```python
from build123d import *

# Parameters (mm, degrees)
SKETCH2_R           = 1.4
SKETCH2_R_2         = 2.5
BOSS_EXTRUDE1_DEPTH = 4
BOSS_EXTRUDE2_START = 16.8
SKETCH3_R           = 4.65
SKETCH3_R_2         = 2.5
BOSS_EXTRUDE2_DEPTH = 16.8
SKETCH5_R           = 4.65
SKETCH5_R_2         = 2.5
BOSS_EXTRUDE3_DEPTH = 2
FILLET1_R           = 2
RIB1_REACH          = 36.514
SKETCH6_WALL_W      = 80.220281068
SKETCH6_WALL_H      = 1.6


with BuildPart() as part:
    # Sketch2 → Boss-Extrude1 (new body)
    with BuildSketch(Plane(origin=(0, 0, 0), x_dir=(1, 0, 0), z_dir=(0, 1, 0))):
        with BuildLine():
            Line((-9.4, -4.65), (0, -4.65))
            ThreePointArc((0, -4.65), (3.288046533, -3.288046533), (4.65, 0))
            Line((4.65, 0), (4.65, 22.6))
            ThreePointArc((4.65, 22.6), (0, 27.25), (-4.65, 22.6))
            Line((-4.65, 22.6), (-4.65, 2.35))
            Line((-4.65, 2.35), (-9.4, 2.35))
            ThreePointArc((-9.4, 2.35), (-12.9, -1.15), (-9.4, -4.65))
        make_face()
        with Locations(Location((-9.4, -1.15, 0), (0, 0, 270))):
            Circle(SKETCH2_R, mode=Mode.SUBTRACT)
        with Locations(Location((0, -1.15, 0), (0, 0, 270))):
            Circle(SKETCH2_R, mode=Mode.SUBTRACT)
        with Locations(Location((0, 22.6, 0), (0, 0, 270))):
            Circle(SKETCH2_R_2, mode=Mode.SUBTRACT)
    extrude(amount=BOSS_EXTRUDE1_DEPTH)

    # Sketch3 → Boss-Extrude2 (add)
    with BuildSketch(Plane.XZ.offset(BOSS_EXTRUDE2_START)):
        with Locations((0, -22.6)):
            Circle(SKETCH3_R)
        with Locations(Location((0, -22.6, 0), (0, 0, 90))):
            Circle(SKETCH3_R_2, mode=Mode.SUBTRACT)
    extrude(amount=-BOSS_EXTRUDE2_DEPTH)

    # Sketch5 → Boss-Extrude3 (add)
    with BuildSketch(Plane(origin=(0, 4, 0), x_dir=(1, 0, 0), z_dir=(0, 1, 0))):
        with Locations(Location((0, 22.6, 0), (0, 0, 270))):
            Circle(SKETCH5_R)
        with Locations(Location((0, 22.6, 0), (0, 0, 270))):
            Circle(SKETCH5_R_2, mode=Mode.SUBTRACT)
    extrude(amount=BOSS_EXTRUDE3_DEPTH)

    # Fillet1
    fillet1_edges = [part.edges().sort_by_distance(p)[0] for p in [
        (0, 6, -27.25),
    ]]
    fillet(fillet1_edges, radius=FILLET1_R - 0.0001)  # a hair under: the kernel refuses the full size

    # Sketch6 wall → Rib1 (add, up to next)
    with BuildSketch(Plane(origin=(0, -3.25, -14.7), x_dir=(0, -0.707106781187, -0.707106781187), z_dir=(0, 0.707106781187, -0.707106781187)), mode=Mode.PRIVATE) as rib1_sk1:
        Rectangle(SKETCH6_WALL_W, SKETCH6_WALL_H)
    rib1_tool1 = extrude(rib1_sk1.sketch, amount=RIB1_REACH, mode=Mode.PRIVATE) - part.part
    add(rib1_tool1.solids().sort_by_distance((0, -3.25, -14.7))[0])


solid = part.part
```
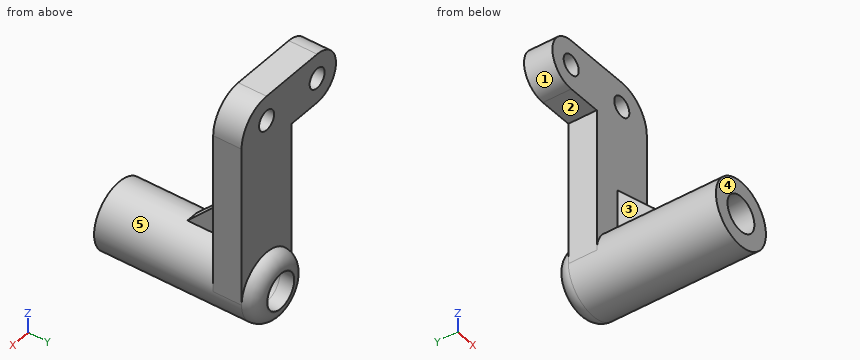
For this review, take the finished solid that the model builds, in its own axes (mm). Face numbers are marked on the shaded views. A direction names the side the tool comes from. Round coordinates to 2 decimals unless told otherwise and drop trailing zeros. Order: outer loops, then holes, each group sorted by start corner. A loop starts at its lowest first (then second) coordinate and runs counter-clockwise, first axis right, second up. Notation, with made-up numbers: (75, 0) -> (94, 0) arc R26 ccw to (94, 17) -> close; hole circle Ø7 at (43.5, 1). An arc over 180 degrees is marked (long way). Use a Markdown table: item, result.
Item 1: For line 1 along X through (y, z) = (1.15, 1.15); line 2 along X through (y, z) = (1.4, -22.6); line 3 along Y through (x, z) = (-3.25, -4.5), list the stretches that pass through material, from the lowest coordinate up. Write a range as [from, to].
Resolved:
| item | result |
|---|---|
| line 1 | x = [-12.9, -10.8], [-8, -1.4], [1.4, 4.51] |
| line 2 | x = [-4.65, -2.5], [2.5, 4.65] |
| line 3 | y = [0, 4] |
Item 2: Take a section at D-D (x = -6.5). State the section outline as (y, z) points.
Resolved:
| item | result |
|---|---|
| outline | (0, -2.35) -> (4, -2.35) -> (4, 4.65) -> (0, 4.65) -> close |
Item 3: For pin 1 (4.5 mm diameter, centred on y = 2.5, z = -16, fed in from -X); pin 2 (5.5 mm diameter, centred on x = -4.5, z = -11, fed in from +Y); pin 3 (9 mm diameter, centred on x = -7, z = -14.5, fed in from -Y), all flat-tipped, find the tip position at first contact; note any pin that passes through.
Resolved:
| item | result |
|---|---|
| pin 1 | stops at x = -4.65 |
| pin 2 | stops at y = 4 |
| pin 3 | stops at y = 0 |
Item 4: Take a section at A-A (z = -15). State the section outline as (x, y) points.
Resolved:
| item | result |
|---|---|
| outline | (-4.65, 0) -> (-0.8, 0) -> (-0.8, -3.55) -> (0.8, -3.55) -> (0.8, 0) -> (4.65, 0) -> (4.65, 4) -> (-4.65, 4) -> close |
Item 5: Take a section at C-C (y = -3.75). State the section outline as (x, z) points.
Resolved:
| item | result |
|---|---|
| outline | (-0.8, -18.02) arc R4.65 ccw (long way) to (0.8, -18.02) -> (0.8, -15.2) -> (-0.8, -15.2) -> close; hole circle Ø5 at (0, -22.6) |
Item 6: Machinability: for the marked faces 1, 2, 3, 4 and 5, which of the approach directions +Z, -Z, +X, -X, +Y, -Y give a long, thin tool a straight path to every point of the face, cutting with its end or side? Answer none if there is none.
Resolved:
| item | result |
|---|---|
| face 1 | -X, +Y, -Y |
| face 2 | -Z, -X, +Y, -Y |
| face 3 | +Z, -X, -Y |
| face 4 | +Z, -Z, +X, -X, -Y |
| face 5 | -Y |
Item 7: Take a section at B-B (y = 1.25). State the section outline as (x, z) points.
Resolved:
| item | result |
|---|---|
| outline | (-9.4, -2.35) -> (-4.65, -2.35) -> (-4.65, -22.6) arc R4.65 ccw to (4.65, -22.6) -> (4.65, 0) arc R4.65 ccw to (0, 4.65) -> (-9.4, 4.65) arc R3.5 ccw to start; hole circle Ø2.8 at (-9.4, 1.15); hole circle Ø5 at (0, -22.6); hole circle Ø2.8 at (0, 1.15) |
